```python
from build123d import *

# Parameters (mm, degrees)
SKETCH1_W           = 60
SKETCH1_H           = 20
BOSS_EXTRUDE1_DEPTH = 2.5
SKETCH2_W           = 60
SKETCH2_H           = 1.66
CUT_EXTRUDE1_DEPTH  = 2
SKETCH3_W           = 1.66
SKETCH3_H           = 18
CUT_EXTRUDE2_DEPTH  = 2
SKETCH4_W           = 58
SKETCH4_H           = 1.66
BOSS_EXTRUDE2_DEPTH = 2
SKETCH5_W           = 1.66
SKETCH5_H           = 20
BOSS_EXTRUDE3_DEPTH = 2


with BuildPart() as part:
    # Sketch1 → Boss-Extrude1 (new, symmetric)
    with BuildSketch(Plane.XY):
        Rectangle(SKETCH1_W, SKETCH1_H)
    extrude(amount=BOSS_EXTRUDE1_DEPTH, both=True)

    # Sketch2 → Cut-Extrude1 (cut)
    with BuildSketch(Plane(origin=(0, 10, 0), x_dir=(1, 0, 0), z_dir=(0, 1, 0))):
        Rectangle(SKETCH2_W, SKETCH2_H)
    extrude(amount=-CUT_EXTRUDE1_DEPTH, mode=Mode.SUBTRACT)

    # Sketch3 → Cut-Extrude2 (cut)
    with BuildSketch(Plane.ZY.offset(30)):
        with Locations((0, -1)):
            Rectangle(SKETCH3_W, SKETCH3_H)
    extrude(amount=-CUT_EXTRUDE2_DEPTH, mode=Mode.SUBTRACT)

    # Sketch4 → Boss-Extrude2 (add)
    with BuildSketch(Plane.XZ.offset(10)):
        with Locations((1, 0)):
            Rectangle(SKETCH4_W, SKETCH4_H)
    extrude(amount=BOSS_EXTRUDE2_DEPTH)

    # Sketch5 → Boss-Extrude3 (add)
    with BuildSketch(Plane(origin=(30, 0, 0), x_dir=(0, 0, -1), z_dir=(1, 0, 0))):
        with Locations((0, -2)):
            Rectangle(SKETCH5_W, SKETCH5_H)
    extrude(amount=BOSS_EXTRUDE3_DEPTH)


solid = part.part
```
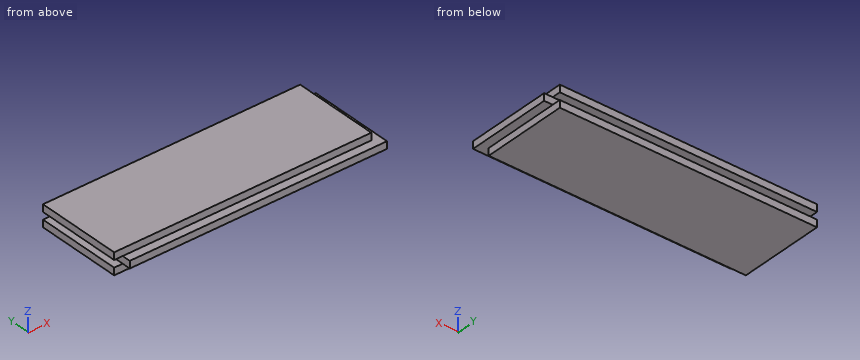
Design review of the part built by this model. Coordinates are the model's own, in mm. Give positions to 0.01 mm unless a question says otherwise; leave off trailing zeros. Order: outer loops, then holes, each group sorted by start corner. A loop starts at its lowest first (then second) coordinate and runs counter-clockwise, first axis right, second up. Notation, with made-up numbers: (72.5, 34.5) - (110.5, 34.5) arc R20 cw to (110.5, 40.5) - close; hole circle Ø1 at (64, 53). An arc over 180 degrees is marked (long way). Use a Markdown table: item, result. Add a question column.
(1) Add section B-B on y = -3. Give the boundary of the cut face in (x, z).
(2) Clearance check with flat-ended pins moving along their axes: P1, Ø0.5, axis at x = 8.5, z = 2, coming from the -Y side; P2, Ø0.5, axis at y = 1.5, z = -1.5, coming from the +X side; P3, Ø0.5, axis at y = -0.5, z = 0, coming from the -X side. State where each tip first meets the part, or that it passes through.
(3) Wall thickness on probe 1 along X at (y, z) = (5.5, 2.25); probe 2 along Y at (x, z) = (-0.5, 0.9); probe 3 along X at (y, z) = (-1.5, 0.7): over which ranges is each line inside the solid? List them lowest first. Write a range as [from, to].
(4) Add section C-C on z = -1.7. Give the boundary of the cut face in (x, y).
(5) Add section A-A on x = 10.5. Give the boundary of the cut face in (y, z).
Report:
| question | item | result |
|---|---|---|
| 1 | outline | (-30, -2.5) - (30, -2.5) - (30, -0.83) - (32, -0.83) - (32, 0.83) - (30, 0.83) - (30, 2.5) - (-30, 2.5) - (-30, 0.83) - (-28, 0.83) - (-28, -0.83) - (-30, -0.83) - close |
| 2 | P1 | stops at y = -10 |
| 2 | P2 | stops at x = 30 |
| 2 | P3 | stops at x = -28 |
| 3 | probe 1 | x = [-30, 30] |
| 3 | probe 2 | y = [-10, 10] |
| 3 | probe 3 | x = [-28, 32] |
| 4 | outline | (-30, -10) - (30, -10) - (30, 10) - (-30, 10) - close |
| 5 | outline | (-12, -0.83) - (-10, -0.83) - (-10, -2.5) - (10, -2.5) - (10, -0.83) - (8, -0.83) - (8, 0.83) - (10, 0.83) - (10, 2.5) - (-10, 2.5) - (-10, 0.83) - (-12, 0.83) - close |
